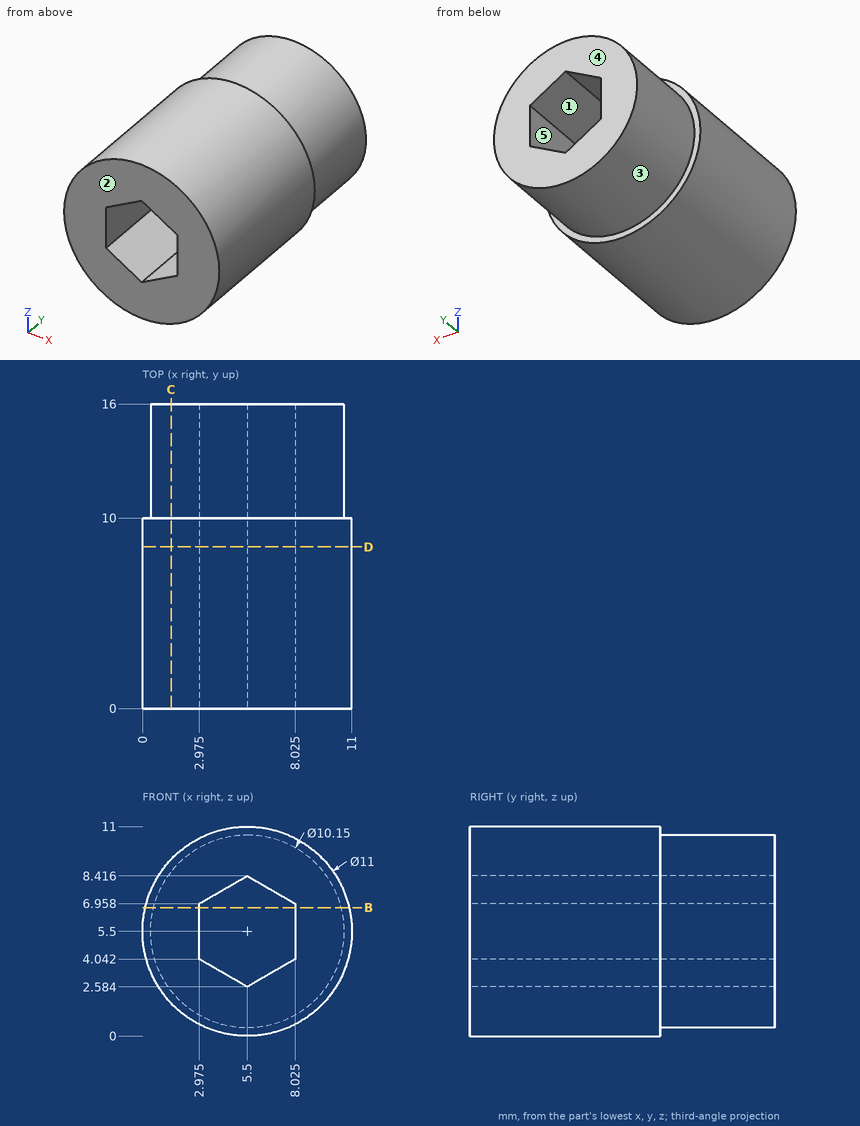
Job drawing, mm, ordinate dimensions from the low corner. One solid piece. A direction names the side the tool comes from. Round coordinates to 2 decimals unless told otherwise and drop trailing zeros. Loops run counter-clockwise (first coordinate to the right, second up) from the corner with the lowest first, then second, coordinate; pieces in that order, holes last. Notation, with made-up numbers: M 26,4 L 43,4 A26 cw 43,30 Z; hole C 7.25,-5.5 d7. An arc over 180 degrees is marked long. Answer as CSV lines item,"result".
1. Cut at C-C on x = 1.5. Write the cut outline in (y, z) (1 decimal), then the cut area to 3 significant figures.
Resolved:
outline,"M 0,1.7 L 10,1.7 L 10,2.4 L 16,2.4 L 16,8.6 L 10,8.6 L 10,9.3 L 0,9.3 Z"
area,"113 mm²"
2. Cut at B-B on z = 6.75. Write the cut outline in (x, y) (1 decimal).
Resolved:
outline,"M 0.1,0 L 3,0 L 3,16 L 0.6,16 L 0.6,10 L 0.1,10 Z; M 8,0 L 10.9,0 L 10.9,10 L 10.4,10 L 10.4,16 L 8,16 Z"
3. Flat gauge pins, fed straight in: P1, Ø3, axis at y = 13.5, z = 6, coming from the +X side (3 decimals); P2, Ø3, axis at y = 11, z = 2, coming from the -X side; P3, Ø1, axis at x = 4, y = 11, coming from the -Z side (1 decimal). Where does each tip first touch, or does it go through?
Resolved:
P1,"stops at x = 10.575"
P2,"stops at x = 0.54"
P3,"stops at z = 0.5"
4. Wall check: probe 1 along Z at (x, y) = (5.25, 1.5) (1 decimal); probe 2 along Z at (x, y) = (7.75, 9.5) (1 decimal); probe 3 along X at (y, z) = (8.75, 6) (1 decimal). Give the ranges that are in metal, low to high. Write a range as [from, to].
Resolved:
probe 1,"z = [0, 2.7], [8.3, 11]"
probe 2,"z = [0.5, 3.9], [7.1, 10.5]"
probe 3,"x = [0, 3], [8, 11]"
5. Cut at D-D on y = 8.5. Write the cut outline in (x, z) (1 decimal).
Resolved:
outline,"C 5.5,5.5 d11; hole M 3,4 L 5.5,2.6 L 8,4 L 8,7 L 5.5,8.4 L 3,7 Z"
6. 3-axis set-ups, long thin cutter, end or side, ignore diameter. For the marked faces 4 and 5: which of +Z, -Z, +X, -X, +Y, -Y reach the whole face in a straight line?
Resolved:
face 4,"+Z, -Z, +X, -X, +Y"
face 5,"+Y, -Y"
7. Two-plate mould, pull along Z, no slides. Class the marked faces 1, 2 and 3: released by +Z, released by -Z, zero draft, split by the parting line, or undercut.
Resolved:
face 1,"undercut"
face 2,"zero draft"
face 3,"split by the parting line"
